```python
from build123d import *

# Parameters (mm, degrees)
F0_R     = 15.920661
F1_DEPTH = 25.4


with BuildPart() as f1:
    # F0 (on Top) → F1 (new body)
    with BuildSketch(Plane.XY):
        with BuildLine():
            ThreePointArc((-46.308367, -28.973528), (-17.604609, 0), (-46.308367, 28.973528))
            ThreePointArc((-46.308367, 28.973528), (-75.554202, 0), (-46.308367, -28.973528))
        make_face()
        with Locations((-46.579406, 0)):
            Circle(F0_R, mode=Mode.SUBTRACT)
        with BuildLine():
            Line((46.842293, 28.102132), (-46.308367, 28.973528))
            ThreePointArc((-46.308367, 28.973528), (-17.604609, 0), (-46.308367, -28.973528))
            Line((-46.308367, -28.973528), (46.842293, -28.102132))
            ThreePointArc((46.842293, -28.102132), (74.682768, 0), (46.842293, 28.102132))
        make_face()
        with Locations((46.579406, 0)):
            Circle(F0_R, mode=Mode.SUBTRACT)
    extrude(amount=F1_DEPTH)


solid = f1.part
```
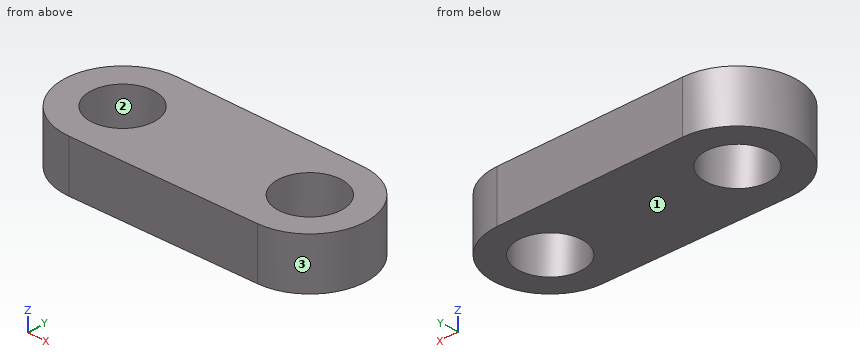
Geometry check sheet. Reference: the model listing, model coordinates, mm. Face numbers are marked on the shaded views. Coordinates: 2 decimals unless noted, no trailing zeros. Order: outer loops, then holes, each group sorted by start corner. A loop starts at its lowest first (then second) coordinate and runs counter-clockwise, first axis right, second up. Notation, with made-up numbers: M 18,-3 L 33,-3 A23 cw 33,36 Z; hole C -25.5,32 d7. An arc over 180 degrees is marked long. Answer as a JSON object with one key per item and string values.
Q1. Cross-section at A-A on y = 0. Record the cut outline in (x, z).
Results are:
{"outline": "M -75.55,0 L -62.5,0 L -62.5,25.4 L -75.55,25.4 Z; M -30.66,0 L 30.66,0 L 30.66,25.4 L -30.66,25.4 Z; M 62.5,0 L 74.68,0 L 74.68,25.4 L 62.5,25.4 Z"}
Q2. Release check for a two-part mould opening along Y. For the marked faces 1, 2 and 3 record: released by +Y, released by -Y, zero draft, split by the parting line, or undercut.
Results are:
{"face 1": "zero draft", "face 2": "undercut", "face 3": "split by the parting line"}
Q3. Depth check by flat-ended pin: pin 1 Ø1 at (x, z) = (40.5, 11.5) entering from -Y; pin 2 Ø1 at (x, z) = (-36, 19.5) entering from -Y; pin 3 Ø10 at (x, z) = (53, 21) entering from -Y. Enter the tip coordinate at first touch or a pass-through.
Results are:
{"pin 1": "stops at y = -28.17", "pin 2": "stops at y = -28.88", "pin 3": "stops at y = -28.07"}
Q4. Cross-section at B-B on z = 4.25. Record the cut outline in (x, y).
Results are:
{"outline": "M -46.31,-28.97 L 46.84,-28.1 A28.1 ccw 46.84,28.1 L -46.31,28.97 A28.97 ccw long Z; hole C -46.58,0 d31.84; hole C 46.58,0 d31.84"}
Q5. Scan lines: line 1 (X direction, y = -8.5, z = 14.5); line 2 (Y direction, x = 47, z = 3.75); line 3 (X direction, y = -7, z = 6). Record each from-to range of solid material in increasing order.
Results are:
{"line 1": "x = -74.28 to -60.04, -33.12 to 33.12, 60.04 to 73.37", "line 2": "y = -28.1 to -15.92, 15.92 to 28.1", "line 3": "x = -74.7 to -60.88, -32.28 to 32.28, 60.88 to 73.8"}
Q6. Cross-section at D-D on x = 23. Record the cut outline in (y, z), and give its area (3 significant figures).
Results are:
{"outline": "M -28.33,0 L 28.33,0 L 28.33,25.4 L -28.33,25.4 Z", "area": "1,440 mm²"}
Q7. Cross-section at C-C on y = 14.5. Record the cut outline in (x, z).
Results are:
{"outline": "M -71.67,0 L -53.15,0 L -53.15,25.4 L -71.67,25.4 Z; M -40.01,0 L 40.01,0 L 40.01,25.4 L -40.01,25.4 Z; M 53.15,0 L 70.65,0 L 70.65,25.4 L 53.15,25.4 Z"}
